```python
from build123d import *

# Parameters (mm, degrees)
EXTRUDE_THIN1_DEPTH = 90
FILLET1_R           = 1
FILLET2_R           = 0.25
FILLET3_RADIUS      = 0.5
FILLET3_LENGTH      = 180
FILLET4_RADIUS      = 0.5
FILLET4_LENGTH      = 180
CUT_EXTRUDE1_DEPTH  = 93.330926563
LPATTERN1_COUNT     = 5
LPATTERN1_PITCH     = 20


with BuildPart() as part:
    # Sketch1 → Extrude-Thin1 (new, symmetric)
    with BuildSketch(Plane.XY):
        Polygon((-20, 5), (-15, 5), (-15, 0), (15, 0), (15, 5), (20, 5), (20, 6), (14, 6), (14, 1), (-14, 1), (-14, 6), (-20, 6), align=None)
    extrude(amount=EXTRUDE_THIN1_DEPTH, both=True)

    # Fillet1
    fillet1_edges = [part.edges().sort_by_distance(p)[0] for p in [
        (-14, 1, 0),
        (14, 1, 0),
    ]]
    fillet(fillet1_edges, radius=FILLET1_R)

    # Fillet2
    fillet2_edges = [part.edges().sort_by_distance(p)[0] for p in [
        (-14, 6, 0),
        (14, 6, 0),
    ]]
    fillet(fillet2_edges, radius=FILLET2_R)

    # Fillet3: full round fillet: the end face becomes a half cylinder, R = half its width
    fillet3_face = Plane((20, 5.5, 0), x_dir=(0, 0, 1), z_dir=(1, 0, 0))  # on the end face: x along it, z out of the body
    fillet3_slab = fillet3_face.offset(-FILLET3_RADIUS / 2) * Box(FILLET3_LENGTH, 2 * FILLET3_RADIUS, FILLET3_RADIUS, mode=Mode.PRIVATE)  # the body's end, R deep
    fillet3_round = Plane((19.5, 5.5, 0), x_dir=(1, 0, 0), z_dir=(0, 0, 1)) * Cylinder(FILLET3_RADIUS, FILLET3_LENGTH, mode=Mode.PRIVATE)  # its axis R under the face
    add(fillet3_slab - fillet3_round, mode=Mode.SUBTRACT)

    # Fillet4: full round fillet: the end face becomes a half cylinder, R = half its width
    fillet4_face = Plane((-20, 5.5, 0), x_dir=(0, 0, 1), z_dir=(-1, 0, 0))  # on the end face: x along it, z out of the body
    fillet4_slab = fillet4_face.offset(-FILLET4_RADIUS / 2) * Box(FILLET4_LENGTH, 2 * FILLET4_RADIUS, FILLET4_RADIUS, mode=Mode.PRIVATE)  # the body's end, R deep
    fillet4_round = Plane((-19.5, 5.5, 0), x_dir=(-1, 0, 0), z_dir=(0, 0, 1)) * Cylinder(FILLET4_RADIUS, FILLET4_LENGTH, mode=Mode.PRIVATE)  # its axis R under the face
    add(fillet4_slab - fillet4_round, mode=Mode.SUBTRACT)

    # Sketch2 → Cut-Extrude1 (cut, through all)
    with BuildSketch(Plane(origin=(0, 1, 0), x_dir=(1, 0, 0), z_dir=(0, 1, 0))):
        with BuildLine():
            Line((-2.5, -5), (-2.5, 5))
            ThreePointArc((-2.5, 5), (0, 7.5), (2.5, 5))
            Line((2.5, 5), (2.5, -5))
            ThreePointArc((2.5, -5), (0, -7.5), (-2.5, -5))
        make_face()
    cut_extrude1 = extrude(amount=-CUT_EXTRUDE1_DEPTH, mode=Mode.SUBTRACT)

    # LPattern1: Cut-Extrude1 ×5
    with Locations(*[(0, 0, -i * LPATTERN1_PITCH) for i in range(1, LPATTERN1_COUNT)]):
        add(cut_extrude1, mode=Mode.SUBTRACT)


solid = part.part
```
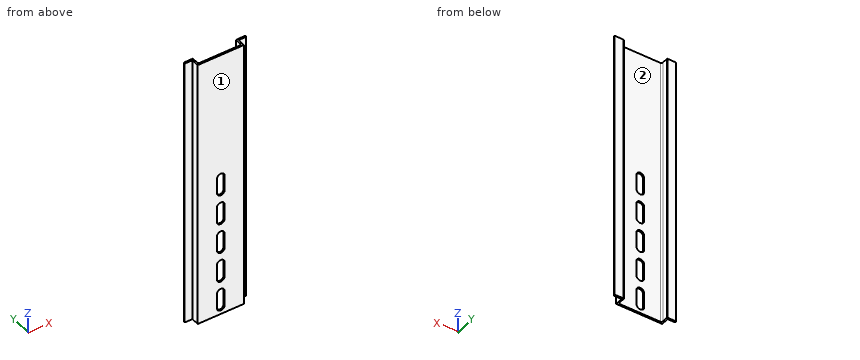
Check sheet for the modelled part. Datum: model origin and axes. Units: mm. Face numbers are marked on the shaded views. Give positions to 0.01 mm unless a question says otherwise; leave off trailing zeros. Loops run counter-clockwise (first coordinate to the right, second up) from the corner with the lowest first, then second, coordinate; pieces in that order, holes last. Notation, with made-up numbers: M 74,69.25 L 124,69.25 A34 cw 124,104.25 Z; hole C 22,-30.5 d10. An arc over 180 degrees is marked long. Answer in a Markdown table with one row per item.
1) Mould release check, pull along X, two halves, no side actions. Record for the marked faces 1 and 2: released by +X, released by -X, zero draft, split by the parting line, or undercut.
Solutions:
| item | result |
|---|---|
| face 1 | zero draft |
| face 2 | undercut |
2) Depth check by flat-ended pin: pin 1 (2 mm diameter, centred on x = 17, z = 3.5, fed in from -Y); pin 2 (1.1 mm diameter, centred on y = 0.5, z = -0.5, fed in from -X); pin 3 (2.5 mm diameter, centred on y = 3.5, z = -43, fed in from +X). Enter the tip coordinate at first touch or a pass-through.
Solutions:
| item | result |
|---|---|
| pin 1 | stops at y = 5 |
| pin 2 | stops at x = -15 |
| pin 3 | stops at x = 15 |
3) Cross-section at C-C (z = 31.5). Enter the section's corners in (x, y), plus the area to 3 significant figures.
Solutions:
| item | result |
|---|---|
| outline | M -19.5,5 L -15,5 L -15,0 L 15,0 L 15,5 L 19.5,5 A0.5 ccw 19.5,6 L 14.25,6 A0.25 ccw 14,5.75 L 14,2 A1 cw 13,1 L -13,1 A1 cw -14,2 L -14,5.75 A0.25 ccw -14.25,6 L -19.5,6 A0.5 ccw Z |
| area | 50.2 mm^2 |
4) Cross-section at B-B (x = 0). Enter the section's corners in (y, z), plus the area to 3 significant figures.
Solutions:
| item | result |
|---|---|
| outline | M 0,-90 L 1,-90 L 1,-87.5 L 0,-87.5 Z; M 0,-72.5 L 1,-72.5 L 1,-67.5 L 0,-67.5 Z; M 0,-52.5 L 1,-52.5 L 1,-47.5 L 0,-47.5 Z; M 0,-32.5 L 1,-32.5 L 1,-27.5 L 0,-27.5 Z; M 0,-12.5 L 1,-12.5 L 1,-7.5 L 0,-7.5 Z; M 0,7.5 L 1,7.5 L 1,90 L 0,90 Z |
| area | 105 mm^2 |
5) Thickness scan on line 1 (X direction, y = 0.3, z = -17.5); line 2 (X direction, y = 3.75, z = 59); line 3 (Y direction, x = 6, z = 32). Record the ranges inside material, lowest first.
Solutions:
| item | result |
|---|---|
| line 1 | x = -15 to -2.5, 2.5 to 15 |
| line 2 | x = -15 to -14, 14 to 15 |
| line 3 | y = 0 to 1 |
6) Cross-section at A-A (z = -22.5). Enter the section's corners in (x, y).
Solutions:
| item | result |
|---|---|
| outline | M -19.5,5 L -15,5 L -15,0 L -2.5,0 L -2.5,1 L -13,1 A1 cw -14,2 L -14,5.75 A0.25 ccw -14.25,6 L -19.5,6 A0.5 ccw Z; M 2.5,0 L 15,0 L 15,5 L 19.5,5 A0.5 ccw 19.5,6 L 14.25,6 A0.25 ccw 14,5.75 L 14,2 A1 cw 13,1 L 2.5,1 Z |
7) Cross-section at D-D (x = -17). Enter the section's corners in (y, z).
Solutions:
| item | result |
|---|---|
| outline | M 5,-90 L 6,-90 L 6,90 L 5,90 Z |
